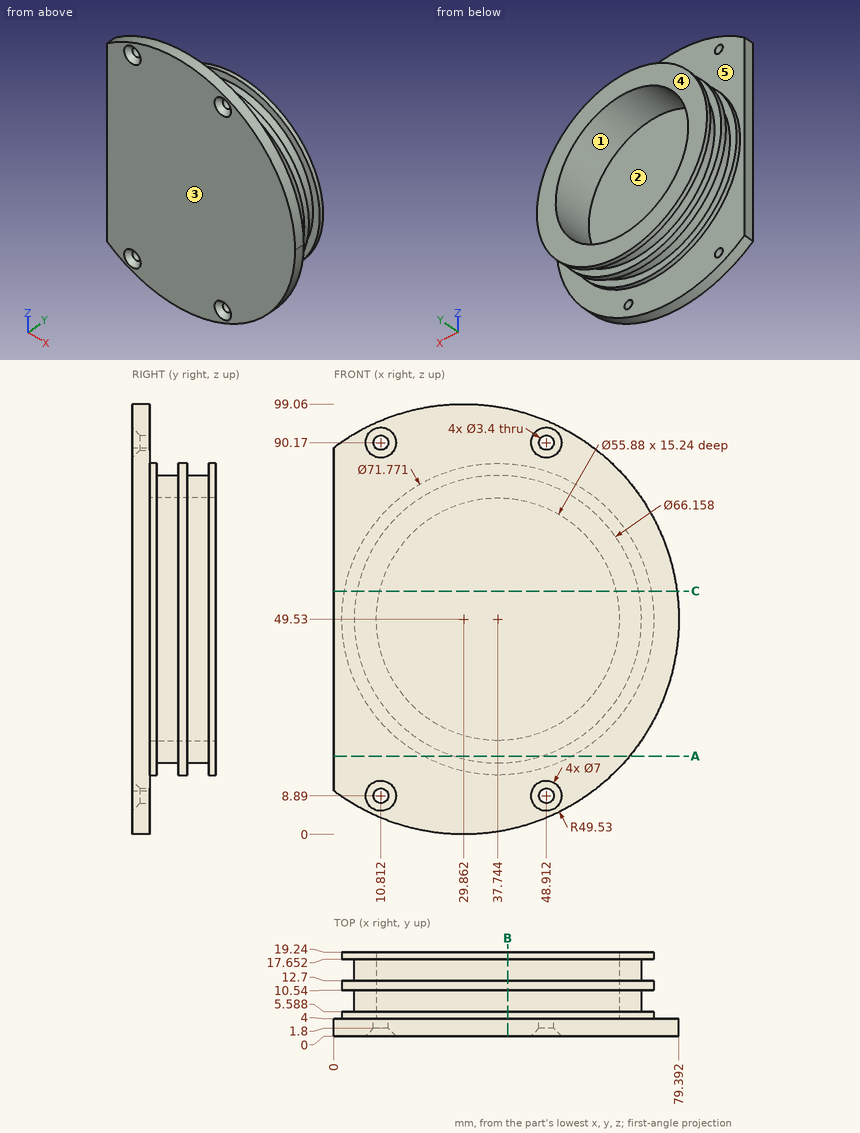
Study the drawing (mm; zero at the part's minimum x, y, z) and answer. A direction names the side the tool comes from. Round coordinates to 2 decimals unless told otherwise and drop trailing zeros. Write each loop counter-clockwise with the first axis right and the second up, starting at its lowest first coordinate (ties: lowest second). Pieces come first, ordered by that corner, then holes.
1) A cutting plane is placed at C-C (z = 56). Give the vertices of the cut face in (x, y) (1 decimal).
2) Straight lines are drawn through the part: line 1 (Y direction, x = 20.5, z = 18.5); line 2 (Z direction, x = 9.5, y = 3.5); line 3 (X direction, y = 17.5, z = 53.5) (1 decimal). For each, find the intervals that lie inside material, in ascending order.
3) Given pin 1 Ø5 at (x, y) = (68, 17) entering from -Z; pin 2 Ø4.5 at (x, z) = (48.91, 90.17) entering from -Y; pin 3 Ø3 at (x, y) = (20.5, 12) entering from +Z, each flat-ended and moving along its own axis, determine where each tip first touches the part or whether it passes through.
4) A cutting plane is placed at B-B (x = 40). Give the vertices of the cut face in (y, z) (1 decimal), plus the area to 3 significant figures.
5) The mould has two halves that part along Z. Classify the marked faces 1, 2 and 3: pulls with the +Z half, pulls with the -Z half, needs draft (parallel to the pull), parting line crosses it, or undercut.
6) A tool of negligible diameter and unlimited length cuts with its end or side. For the marked faces 4 and 5, from which of +Z, -Z, +X, -X, +Y, -Y can it reach the whole face along a straight path? Write none if from no direction.
7) A cutting plane is placed at A-A (z = 18). Give the vertices of the cut face in (x, y).
Completed:
1. outline: (0, 0) - (79, 0) - (79, 4) - (73, 4) - (73, 5.6) - (70.2, 5.6) - (70.2, 10.5) - (73, 10.5) - (73, 12.7) - (70.2, 12.7) - (70.2, 17.7) - (73, 17.7) - (73, 19.2) - (64.9, 19.2) - (64.9, 4) - (10.6, 4) - (10.6, 19.2) - (2.4, 19.2) - (2.4, 17.7) - (5.3, 17.7) - (5.3, 12.7) - (2.4, 12.7) - (2.4, 10.5) - (5.3, 10.5) - (5.3, 5.6) - (2.4, 5.6) - (2.4, 4) - (0, 4) - close
2. line 1: y = 0 to 5.59, 10.54 to 12.7, 17.65 to 19.24
2. line 2: z = 4.38 to 7.81, 9.97 to 89.09, 91.25 to 94.68
2. line 3: x = 4.9 to 10.1, 65.4 to 70.6
3. pin 1: stops at z = 26.89
3. pin 2: stops at y = 1.25
3. pin 3: stops at z = 81.78
4. outline: (0, 1) - (4, 1) - (4, 13.7) - (5.6, 13.7) - (5.6, 16.5) - (10.5, 16.5) - (10.5, 13.7) - (12.7, 13.7) - (12.7, 16.5) - (17.7, 16.5) - (17.7, 13.7) - (19.2, 13.7) - (19.2, 21.7) - (4, 21.7) - (4, 77.4) - (19.2, 77.4) - (19.2, 85.3) - (17.7, 85.3) - (17.7, 82.5) - (12.7, 82.5) - (12.7, 85.3) - (10.5, 85.3) - (10.5, 82.5) - (5.6, 82.5) - (5.6, 85.3) - (4, 85.3) - (4, 98) - (0, 98) - close
4. area: 575 mm2
5. face 1: undercut
5. face 2: undercut
5. face 3: needs draft
6. face 4: +Z, -Z, +X, -X, +Y
6. face 5: +Y
7. outline: (0, 0) - (68.06, 0) - (68.06, 4) - (54.88, 4) - (54.88, 5.59) - (47.75, 5.59) - (47.75, 10.54) - (54.88, 10.54) - (54.88, 12.7) - (47.75, 12.7) - (47.75, 17.65) - (54.88, 17.65) - (54.88, 19.24) - (20.61, 19.24) - (20.61, 17.65) - (27.74, 17.65) - (27.74, 12.7) - (20.61, 12.7) - (20.61, 10.54) - (27.74, 10.54) - (27.74, 5.59) - (20.61, 5.59) - (20.61, 4) - (0, 4) - close
